Geometry check sheet. Reference: the model listing, model coordinates, mm. A direction names the side the tool comes from. Give positions to 0.01 mm unless a question says otherwise; leave off trailing zeros. Loops run counter-clockwise (first coordinate to the right, second up) from the corner with the lowest first, then second, coordinate; pieces in that order, holes last.
1. Go/stop test with a flat-tipped pin: pin 1 Ø1 at (x, y) = (45.5, 17) entering from +Z. Record where the tip stops, or that it passes through.
2. Cross-section at C-C, the plane y = 9. Record the cut outline in (x, z) (1 decimal).
3. Cross-section at D-D, the plane x = 45. Record the cut outline in (y, z) (1 decimal).
4. Material ranges on L1, parallel to X at y = 7.5, z = 2.85 (3 decimals); L2, parallel to Y at x = 42, z = 2.25 (3 decimals); L3, parallel to X at y = 12.75, z = 0.3, recorded low to high.
5. Cross-section at B-B, the plane z = 0.95. Record the cut outline in (x, y) (1 decimal).
6. Tool access check on faces 4 (the flat face through (25, 13, 0)), 5 (the flat face through (25, 3.175, 2)). Record the directions out of +Z, -Z, +X, -X, +Y, -Y that give a thin tool (end or side, any length) a straight path to the whole face; none if there is none.
7. Cross-section at A-A, the plane y = 12.7. Record the cut outline in (x, z) (1 decimal), plus the area to 3 significant figures.
8. Release check for a two-part mould opening along Y. For faces 1 (the cylindrical face through (49.272, 1.449, 1.61)), 2 (the flat face through (25, 22.225, 2)), 3 (the flat face through (25, 2, 3.175)) record: +Y half, -Y half, draft (parallel to the pull), parting line (faces both ways), or undercut.
from build123d import *

# Parameters (mm, degrees)
F0_W     = 44.45
F0_H     = 19.05
F0_R     = 2.38125
F1_DEPTH = 1.5875
F0_W_2   = 50.8
F0_H_2   = 25.4
F2_DEPTH = 3.175
F3_R     = 5.08


with BuildPart() as f1:
    # F0 (on Top) → F1 (new body)
    with BuildSketch(Plane.XY):
        with Locations((25.4, 12.7)):
            Rectangle(F0_W, F0_H)
        with Locations((7.14375, 12.7)):
            Circle(F0_R, mode=Mode.SUBTRACT)
    extrude(amount=F1_DEPTH)

    # F0 (on Top) → F2 (join)
    with BuildSketch(Plane.XY):
        with Locations((25.4, 12.7)):
            Rectangle(F0_W_2, F0_H_2)
        with Locations((25.4, 12.7)):
            Rectangle(F0_W, F0_H, mode=Mode.SUBTRACT)
    extrude(amount=F2_DEPTH)

    # F3
    f3_edges = [f1.edges().sort_by_distance(p)[0] for p in [
        (50.8, 0, 1.5875),
        (50.8, 25.4, 1.5875),
        (0, 0, 1.5875),
        (0, 25.4, 1.5875),
    ]]
    fillet(f3_edges, radius=F3_R)


solid = f1.part
Result:
1. pin 1: stops at z = 1.59
2. outline: (0, 0) - (50.8, 0) - (50.8, 3.2) - (47.6, 3.2) - (47.6, 1.6) - (3.2, 1.6) - (3.2, 3.2) - (0, 3.2) - close
3. outline: (0, 0) - (25.4, 0) - (25.4, 3.2) - (22.2, 3.2) - (22.2, 1.6) - (3.2, 1.6) - (3.2, 3.2) - (0, 3.2) - close
4. L1: x = 0 to 3.175, 47.625 to 50.8
4. L2: y = 0 to 3.175, 22.225 to 25.4
4. L3: x = 0 to 4.76, 9.52 to 50.8
5. outline: (0, 5.1) arc R5.1 ccw to (5.1, 0) - (45.7, 0) arc R5.1 ccw to (50.8, 5.1) - (50.8, 20.3) arc R5.1 ccw to (45.7, 25.4) - (5.1, 25.4) arc R5.1 ccw to (0, 20.3) - close; hole circle Ø4.8 at (7.1, 12.7)
6. face 4: -Z, +X, -X, +Y, -Y
6. face 5: +Z
7. outline: (0, 0) - (4.8, 0) - (4.8, 1.6) - (3.2, 1.6) - (3.2, 3.2) - (0, 3.2) - close; (9.5, 0) - (50.8, 0) - (50.8, 3.2) - (47.6, 3.2) - (47.6, 1.6) - (9.5, 1.6) - close
7. area: 83.2 mm2
8. face 1: -Y half
8. face 2: undercut
8. face 3: draft
